The model under review builds one solid part; all positions refer to its coordinate system, in mm. A direction names the side the tool comes from. Round coordinates to 2 decimals unless told otherwise and drop trailing zeros. Order: outer loops, then holes, each group sorted by start corner. A loop starts at its lowest first (then second) coordinate and runs counter-clockwise, first axis right, second up. Notation, with made-up numbers: (50, 67.25) -> (79, 67.25) arc R23 cw to (79, 105.25) -> close; hole circle Ø10 at (79, 15.5). An arc over 180 degrees is marked (long way). Use a Markdown table: item, result. Add a question column.
Autodesk Fusion 360 part; units mm, degrees
sketch "Sketch1" plane through (0, 0, 0) normal (0, 1, 0) x (1, 0, 0)
  line L0 (0, 0) -> (60, 0)
  line L1 (60, 0) -> (60, -7)
  line L2 (60, -7) -> (0, -7)
  line L3 (0, -7) -> (0, 0)
  line L4 (0, -7) -> (2.5, -7)
  line L5 (2.5, -7) -> (2.5, -3.5)
  line L6 (2.5, -3.5) -> (0, -3.5)
  line L7 (0, -3.5) -> (0, -7)
  line L8 (60, -7) -> (57.5, -7)
  line L9 (57.5, -7) -> (57.5, -3.5)
  line L10 (57.5, -3.5) -> (60, -3.5)
  line L11 (60, -3.5) -> (60, -7)
  circle A0 centre (2.5, -3.5) radius 1.25
  circle A1 centre (57.5, -3.5) radius 1.25
  line L12 (0, -7) -> (30, -7)
  line L13 (0, -7) -> (18, -7)
  line L14 (60, -7) -> (42, -7)
  line L15 (2.5, -3.5) -> (7.5, -3.5)
  line L16 (57.5, -3.5) -> (52.5, -3.5)
  circle A2 centre (7.5, -3.5) radius 1.25
  circle A3 centre (52.5, -3.5) radius 1.25
  circle A4 centre (52.5, -3.5) radius 2.5
  circle A5 centre (7.5, -3.5) radius 2.5
  line L17 (7.5, -3.5) -> (15, -3.5)
  line L18 (52.5, -3.5) -> (45, -3.5)
  line L19 (15, -3.5) -> (25, -3.5)
  line L20 (25, -3.5) -> (35, -3.5)
  line L21 (35, -3.5) -> (45, -3.5)
  circle A6 centre (15, -3.5) radius 2
  circle A7 centre (25, -3.5) radius 2
  circle A8 centre (35, -3.5) radius 2
  circle A9 centre (45, -3.5) radius 2
  dimension "d1" = 60
  dimension "d2" = 7
  dimension "d3" = 2.5
  dimension "d4" = 3.5
  dimension "d5" = 2.5
  dimension "d6" = 3.5
  dimension "d7" = 2.5
  dimension "d8" = 2.5
  dimension "d79" = 5
  dimension "d80" = 5
  dimension "d81" = 2.5
  dimension "d82" = 2.5
  dimension "d83" = 5
  dimension "d84" = 5
  dimension "d85" = 7.5
  dimension "d86" = 7.5
  dimension "d87" = 10
  dimension "d88" = 10
  dimension "d89" = 10
  dimension "d90" = 4
  dimension "d91" = 4
  dimension "d92" = 4
  dimension "d93" = 4
extrude "Extrude1" add sketch "Sketch1" along normal blind 3.532 contours L0 L1 L3 L6 L10 A0 A1 L15 L16 A4 A5 L17 L18 L19 L20 L21 A6 A7 A8 A9 | L2 L3 L4 L5 L6 L7 A0 L12 L13 | L1 L2 L8 L9 L10 L11 A1 L14 | L6 A0 L15 | L5 L6 A0 | L9 L10 A1 | L10 A1 L16 | L2 L5 L9 A0 A1 L12 L13 L14 L15 L16 A4 A5 L17 L18 L19 L20 L21 A6 A7 A8 A9 | L5 A0 L15 | L9 A1 L16 | L15 A2 A5 L17 | L15 A2 A5 L17 | L16 A3 A4 L18 | L16 A3 A4 L18 | L15 A2 L17 | L15 A2 L17 | L16 A3 L18 | L16 A3 L18
extrude "Extrude3" cut sketch "Sketch1" along normal blind 2 contours L6 A0 L15 | L5 L6 A0 | L9 L10 A1 | L10 A1 L16 | L5 A0 L15 | L9 A1 L16
extrude "Extrude4" add sketch "Sketch1" against normal blind 1 contours L15 A2 A5 L17 | L15 A2 A5 L17 | L16 A3 A4 L18 | L16 A3 A4 L18
extrude "Extrude12" cut 2 faces at (52.6522, 0, 3.8879) (7.2402, 0, 3.8258) along direction (0, 1, 0) blind 2
sketch "Sketch5" plane through (0, 0, 0) normal (0, -1, 0) x (1, 0, 0)
  circle A0 centre (7.5, 3.5) radius 2.5
  circle A1 centre (2.5, 3.5) radius 1.25
  circle A2 centre (57.5, 3.5) radius 1.25
  circle A3 centre (15, 3.5) radius 2
  circle A4 centre (45, 3.5) radius 2
  circle A5 centre (25, 3.5) radius 2
  circle A6 centre (35, 3.5) radius 2
  line L0 (0, 7) -> (0, 0)
  line L1 (0, 0) -> (60, 0)
  line L2 (60, 0) -> (60, 7)
  line L3 (60, 7) -> (0, 7)
  circle A7 centre (52.5, 3.5) radius 2.5
  line L4 (10, 3.5) -> (10, 7)
  line L5 (10, 7) -> (50, 7)
  line L6 (50, 7) -> (50, 0)
  line L7 (50, 0) -> (10, 0)
  line L8 (10, 0) -> (10, 7)
  line L9 (10, 7) -> (50, 7)
  line L10 (50, 7) -> (50, 6)
  line L11 (50, 6) -> (10, 6)
  line L12 (10, 6) -> (10, 7)
  line L13 (10, 0) -> (50, 0)
  line L14 (50, 0) -> (50, 1)
  line L15 (50, 1) -> (10, 1)
  line L16 (10, 1) -> (10, 0)
  dimension "d94" = 1
extrude "Extrude11" cut sketch "Sketch5" against normal blind 2.7 contours L4 L6 L8 L11 L15
fillet "Fillet4" radius 1 2 edges at (30, 0, 6) (30, 0, 1)
Q1. Wall thickness on line 1 (X direction, y = 1.05, z = 3.5); line 2 (Z direction, x = 18.5, y = 2.6); line 3 (X direction, y = 0.7, z = 5.75): over which ranges is each line inside the solid? List them lowest first. Write a range as [from, to].
Q2. Mouldability with a two-part tool opening along X and no side actions: class faces 1 (the cylindrical face through (6.25, 0.52, 3.45)), 2 (the flat face through (30, 2, 0)), 3 (the flat face through (60, 2, 3)) as pulls with the +X half, pulls with the -X half, needs draft (parallel to the pull), parting line crosses it, or undercut.
Q3. Add section C-C (x = 57.5). Write out the cut boundary in (y, z).
Q4. Add section D-D (z = 0.5). Write out the cut boundary in (x, y).
Q5. Machinability: for faces 4 (the cylindrical face through (54.81, -0.49, 4.46)), 5 (the cylindrical face through (13.002, 3.11, 3.588)), which of the approach directions +Z, -Z, +X, -X, +Y, -Y give a long, thin tool a straight path to every point of the face, cutting with its end or side? Answer none if there is none.
Q6. Insertion check: pin 1 (2 mm diameter, centred on x = 43, z = 3, fed in from -Y); pin 2 (3 mm diameter, centred on x = 57.5, z = 4, fed in from -Y); pin 3 (1.5 mm diameter, centred on x = 7.5, z = 3.5, fed in from -Y). Each pin has a flat end and moves straight along its axis. Give the tip position at first contact, or say it passes through.
Q7. Add section B-B (y = -0.5). Write out the cut boundary in (x, z), then the cut area to 3 significant figures.
Report:
| question | item | result |
|---|---|---|
| 1 | line 1 | x = [0, 1.25], [3.75, 6.25], [8.75, 10], [50, 51.25], [53.75, 56.25], [58.75, 60] |
| 1 | line 2 | z = [0, 1], [6, 7] |
| 1 | line 3 | x = [0, 10], [50, 60] |
| 2 | face 1 | undercut |
| 2 | face 2 | needs draft |
| 2 | face 3 | pulls with the +X half |
| 3 | outline | (0, 0) -> (3.53, 0) -> (3.53, 7) -> (0, 7) -> (0, 4.75) -> (2, 4.75) -> (2, 2.25) -> (0, 2.25) -> close |
| 4 | outline | (0, 0) -> (10, 0) -> (10, 0.13) -> (50, 0.13) -> (50, 0) -> (60, 0) -> (60, 3.53) -> (0, 3.53) -> close |
| 5 | face 4 | -Y |
| 5 | face 5 | +Y, -Y |
| 6 | pin 1 | stops at y = 2.7 |
| 6 | pin 2 | stops at y = 0 |
| 6 | pin 3 | stops at y = 2 |
| 7 | outline | circle Ø5 at (7.5, 3.5); circle Ø5 at (52.5, 3.5); hole circle Ø2.5 at (7.5, 3.5); hole circle Ø2.5 at (52.5, 3.5) |
| 7 | area | 29.5 mm² |
